from build123d import *

# Parameters (mm, degrees)
SKETCH_1_W          = 130
SKETCH_1_H          = 130
SKETCH_1_R          = 1.6
EXTRUDE_1_DEPTH     = 25
SKETCH_2_R          = 5
EXTRUDE_2_DEPTH     = 5
SKETCH_3_R          = 1.5
SKETCH_3_R_2        = 2
CUT_EXTRUDE_1_DEPTH = 103.102889283
FILLET_1_R          = 10
SKETCH_4_R          = 1.6
CUT_EXTRUDE_2_DEPTH = 10
CUT_EXTRUDE_START   = -10
SKETCH_5_R          = 12.5
CUT_EXTRUDE_3_DEPTH = 10
SKETCH_6_OUTSIDE_W  = 169.108
SKETCH_6_OUTSIDE_H  = 169.108
CUT_EXTRUDE_4_DEPTH = 103.102889283
SKETCH_7_R          = 3.5
CUT_EXTRUDE_5_DEPTH = 3
SKETCH_9_R          = 3.5
CUT_EXTRUDE_6_DEPTH = 5
EXTRUDE_START       = -20
SKETCH_10_R         = 1.6
EXTRUDE_3_DEPTH     = 20
EXTRUDE_START_2     = -13
SKETCH_11_R         = 1.5
EXTRUDE_4_DEPTH     = 13


with BuildPart() as part:
    # 草图1 → 凸台-拉伸1 (new body)
    with BuildSketch(Plane(origin=(0, 0, 0), x_dir=(1, 0, 0), z_dir=(0, 1, 0))):
        with Locations((5, 5)):
            Rectangle(SKETCH_1_W, SKETCH_1_H)
        with Locations(Location((61.920310217, 0, 0), (0, 0, 270))):
            Circle(SKETCH_1_R, mode=Mode.SUBTRACT)
        with Locations(Location((40, -21.920310217, 0), (0, 0, 270))):
            Circle(SKETCH_1_R, mode=Mode.SUBTRACT)
        with Locations(Location((40, 21.920310217, 0), (0, 0, 270))):
            Circle(SKETCH_1_R, mode=Mode.SUBTRACT)
        with Locations(Location((21.920310217, 40, 0), (0, 0, 270))):
            Circle(SKETCH_1_R, mode=Mode.SUBTRACT)
        with Locations(Location((-21.920310217, 40, 0), (0, 0, 270))):
            Circle(SKETCH_1_R, mode=Mode.SUBTRACT)
        with Locations(Location((0, 61.920310217, 0), (0, 0, 270))):
            Circle(SKETCH_1_R, mode=Mode.SUBTRACT)
        with BuildLine():
            ThreePointArc((-8.926785536, 31.25), (-22.980970389, -22.980970389), (31.25, -8.926785536))
            ThreePointArc((31.25, -8.926785536), (52.5, 0), (31.25, 8.926785536))
            ThreePointArc((31.25, 8.926785536), (22.980970389, 22.980970389), (8.926785536, 31.25))
            ThreePointArc((8.926785536, 31.25), (0, 52.5), (-8.926785536, 31.25))
        make_face(mode=Mode.SUBTRACT)
    extrude(amount=EXTRUDE_1_DEPTH)

    # 草图2 → 凸台-拉伸2 (add)
    with BuildSketch(Plane.XZ):
        with BuildLine():
            ThreePointArc((-8.926785536, -31.25), (0, -52.5), (8.926785536, -31.25))
            ThreePointArc((8.926785536, -31.25), (22.980970389, -22.980970389), (31.25, -8.926785536))
            ThreePointArc((31.25, -8.926785536), (52.5, 0), (31.25, 8.926785536))
            ThreePointArc((31.25, 8.926785536), (-22.980970389, 22.980970389), (-8.926785536, -31.25))
        make_face()
        with Locations(Location((-20, 0, 0), (0, 0, 270))):
            Circle(SKETCH_2_R, mode=Mode.SUBTRACT)
    extrude(amount=-EXTRUDE_2_DEPTH)

    # 草图3 → 切除-拉伸1 (cut, through all)
    with BuildSketch(Plane(origin=(0, 25, 0), x_dir=(1, 0, 0), z_dir=(0, 1, 0))):
        with Locations(Location((-25, 25, 0), (0, 0, 270))):
            Circle(SKETCH_3_R)
        with Locations(Location((25, 25, 0), (0, 0, 270))):
            Circle(SKETCH_3_R)
        with Locations(Location((-25, -25, 0), (0, 0, 270))):
            Circle(SKETCH_3_R)
        with Locations(Location((25, -25, 0), (0, 0, 270))):
            Circle(SKETCH_3_R)
        with Locations(Location((-45, 45, 0), (0, 0, 270))):
            Circle(SKETCH_3_R_2)
        with Locations(Location((45, 45, 0), (0, 0, 270))):
            Circle(SKETCH_3_R_2)
        with Locations(Location((45, -45, 0), (0, 0, 270))):
            Circle(SKETCH_3_R_2)
        with Locations(Location((-45, -45, 0), (0, 0, 270))):
            Circle(SKETCH_3_R_2)
    extrude(amount=-CUT_EXTRUDE_1_DEPTH, mode=Mode.SUBTRACT)

    # 圆角1
    fillet_1_edges = [part.edges().sort_by_distance(p)[0] for p in [
        (-60, 12.5, -70),
        (70, 12.5, -70),
        (70, 12.5, 60),
        (-60, 12.5, 60),
    ]]
    fillet(fillet_1_edges, radius=FILLET_1_R)

    # 草图4 → 切除-拉伸2 (cut)
    with BuildSketch(Plane(origin=(0, 5, 0), x_dir=(1, 0, 0), z_dir=(0, 1, 0))):
        with Locations(Location((0, 0, 0), (0, 0, 270))):
            Circle(SKETCH_4_R)
    extrude(amount=-CUT_EXTRUDE_2_DEPTH, mode=Mode.SUBTRACT)

    # 草图5 → 切除-拉伸3 (cut)
    with BuildSketch(Plane(origin=(0, 5, 0), x_dir=(1, 0, 0), z_dir=(0, 1, 0)).offset(CUT_EXTRUDE_START)):
        with Locations(Location((40, 0, 0), (0, 0, 134.427004001))):
            Circle(SKETCH_5_R)
        with Locations(Location((0, 40, 0), (0, 0, 315.572995999))):
            Circle(SKETCH_5_R)
    extrude(amount=CUT_EXTRUDE_3_DEPTH, mode=Mode.SUBTRACT)

    # 草图6 outside → 切除-拉伸4 (cut, through all)
    with BuildSketch(Plane(origin=(0, 25, 0), x_dir=(1, 0, 0), z_dir=(0, 1, 0))):
        with Locations((5, 5)):
            Rectangle(SKETCH_6_OUTSIDE_W, SKETCH_6_OUTSIDE_H)
        with BuildLine():
            Line((45, -55), (-45, -55))
            ThreePointArc((-45, -55), (-52.071067812, -52.071067812), (-55, -45))
            Line((-55, -45), (-55, 45))
            ThreePointArc((-55, 45), (-52.071067812, 52.071067812), (-45, 55))
            Line((-45, 55), (45, 55))
            ThreePointArc((45, 55), (52.071067812, 52.071067812), (55, 45))
            Line((55, 45), (55, -45))
            ThreePointArc((55, -45), (52.071067812, -52.071067812), (45, -55))
        make_face(mode=Mode.SUBTRACT)
    extrude(amount=-CUT_EXTRUDE_4_DEPTH, mode=Mode.SUBTRACT)

    # 草图7 → 切除-拉伸5 (cut)
    with BuildSketch(Plane.XZ):
        with Locations(Location((0, 0, 0), (0, 0, 270))):
            Circle(SKETCH_7_R)
    extrude(amount=-CUT_EXTRUDE_5_DEPTH, mode=Mode.SUBTRACT)

    # 草图9 → 切除-拉伸6 (cut)
    with BuildSketch(Plane.XZ):
        with Locations(Location((-21.920310217, -40, 0), (0, 0, 270))):
            Circle(SKETCH_9_R)
        with Locations(Location((21.920310217, -40, 0), (0, 0, 270))):
            Circle(SKETCH_9_R)
        with Locations(Location((40, -21.920310217, 0), (0, 0, 270))):
            Circle(SKETCH_9_R)
        with Locations(Location((40, 21.920310217, 0), (0, 0, 270))):
            Circle(SKETCH_9_R)
        with Locations(Location((-47, 25, 0), (0, 0, 270))):
            Circle(SKETCH_9_R)
        with Locations(Location((-47, -25, 0), (0, 0, 270))):
            Circle(SKETCH_9_R)
    extrude(amount=-CUT_EXTRUDE_6_DEPTH, mode=Mode.SUBTRACT)

    # 草图10 → 凸台-拉伸3 (add)
    with BuildSketch(Plane(origin=(0, 25, 0), x_dir=(1, 0, 0), z_dir=(0, 1, 0)).offset(EXTRUDE_START)):
        with Locations((40, 21.920310217)):
            Circle(SKETCH_10_R)
        with Locations((40, -21.920310217)):
            Circle(SKETCH_10_R)
        with Locations((-21.920310217, 40)):
            Circle(SKETCH_10_R)
        with Locations((21.920310217, 40)):
            Circle(SKETCH_10_R)
    extrude(amount=EXTRUDE_3_DEPTH)

    # 草图11 → 凸台-拉伸4 (add)
    with BuildSketch(Plane.XZ.offset(EXTRUDE_START_2)):
        with Locations(Location((25, 25, 0), (0, 0, 90))):
            Circle(SKETCH_11_R)
        with Locations(Location((-25, 25, 0), (0, 0, 90))):
            Circle(SKETCH_11_R)
        with Locations(Location((-25, -25, 0), (0, 0, 90))):
            Circle(SKETCH_11_R)
        with Locations(Location((25, -25, 0), (0, 0, 90))):
            Circle(SKETCH_11_R)
    extrude(amount=EXTRUDE_4_DEPTH)


solid = part.part
Could you check a few things on this model? Use its own coordinates, in mm. A direction names the side the tool comes from. Round coordinates to 2 decimals unless told otherwise and drop trailing zeros. Order: outer loops, then holes, each group sorted by start corner. A loop starts at its lowest first (then second) coordinate and runs counter-clockwise, first axis right, second up. Notation, with made-up numbers: M 16,41 L 37,41 A31 ccw 37,67 Z; hole C -14.75,20.25 d7. An arc over 180 degrees is marked long. One line per item, written item: value.
(1) I'm going to push flat-ended pins straight in: P1, Ø16, axis at x = -20, z = 0, coming from the -Y side; P2, Ø1, axis at x = 5.5, z = 18.5, coming from the +Y side; P3, Ø2, axis at x = -23, z = -40, coming from the -Y side; P4, Ø1.5, axis at x = 25.5, z = -24.5, coming from the +Y side. Where does each tip first touch, or does it pass through?
Ans:
P1: stops at y = 0
P2: stops at y = 5
P3: stops at y = 5
P4: stops at y = 13
(2) Imagine slicing it at D-D (y = 18.75). Count the separate pieces of the cut face and the enclosed holes in it, and give its area (3 significant figures).
Ans:
separate pieces: 1
enclosed holes: 9
area: 7,760 mm^2
(3) Imagine slicing it at C-C (y = 7.75). Write out the boundary of the cut face in (x, z).
Ans:
outline: M -55,-45 A10 ccw -45,-55 L 45,-55 A10 ccw 55,-45 L 55,45 A10 ccw 45,55 L -45,55 A10 ccw -55,45 Z; hole C -45,-45 d4; hole C -45,45 d4; hole M -8.93,-31.25 A12.5 ccw long 8.93,-31.25 A32.5 ccw 31.25,-8.93 A12.5 ccw long 31.25,8.93 A32.5 ccw long Z; hole C 45,-45 d4; hole C 45,45 d4
(4) Imagine slicing it at B-B (x = 40). Write out the boundary of the cut face in (y, z).
Ans:
outline: M 0,-55 L 25,-55 L 25,-12.5 L 0,-12.5 L 0,-18.42 L 5,-18.42 L 5,-25.42 L 0,-25.42 Z; M 0,12.5 L 25,12.5 L 25,55 L 0,55 L 0,25.42 L 5,25.42 L 5,18.42 L 0,18.42 Z
(5) Which directions (+Z, -Z, +X, -X, +Y, -Y) give clear straight access to the entire face, cutting with the end or side of a thin tool? Please do faces 4 (the cylindrical face through (-47, 13, 45)), 5 (the flat face through (25, 13, -25)), 6 (the flat face through (-47, 5, -25)).
Ans:
face 4: +Y, -Y
face 5: +Y
face 6: -Y
(6) Imagine slicing it at A-A (x = 0). Write out the boundary of the cut face in (y, z).
Ans:
outline: M 0,-55 L 25,-55 L 25,-52.5 L 0,-52.5 Z; M 0,-27.5 L 5,-27.5 L 5,-1.6 L 3,-1.6 L 3,-3.5 L 0,-3.5 Z; M 0,3.5 L 3,3.5 L 3,1.6 L 5,1.6 L 5,32.5 L 25,32.5 L 25,55 L 0,55 Z
(7) I need wall thicknesses on line 1 along X through (y, z) = (3.85, 0); line 2 along X through (y, z) = (2.05, -40); line 3 along Z through (x, y) = (0, 12.75). Which ranges of each line are inside material? Lowest first, please. Write a range as from..to.
Ans:
line 1: x = -55..-25, -15..-1.6, 1.6..27.5, 52.5..55
line 2: x = -55..-25.42, -18.42..-12.5, 12.5..18.42, 25.42..55
line 3: z = -55..-52.5, 32.5..55
(8) If we mould it in two halves opening along Z, with no side actions, what happens to faces 1 (the flat face through (-1, 25, 36)), 2 (the cylindrical face through (-43.53, 2.46, -24.54)), 3 (the cylindrical face through (51.99, 12.68, -52.15))? For each: released by +Z, released by -Z, zero draft, split by the parting line, or undercut.
Ans:
face 1: zero draft
face 2: undercut
face 3: released by -Z
